Autodesk Inventor part; units mm, degrees
ref_plane "YZ Plane" through (0, 0, 0) normal (1, 0, 0) x (0, 1, 0)
ref_plane "XZ Plane" through (0, 0, 0) normal (0, 1, 0) x (-1, 0, 0)
ref_plane "XY Plane" through (0, 0, 0) normal (0, 0, 1) x (1, 0, 0)
sketch "Sketch1" plane through (0, 0, 0) normal (0, 0, 1) x (1, 0, 0)
  line L0 (0, 0) -> (90, 0)
  line L1 (90, 0) -> (90, 60)
  line L2 (90, 60) -> (0, 60)
  line L3 (0, 60) -> (0, 0)
  line L4 (-10, 30) -> (100, 30)
  line L5 (8, 10) -> (8, 50)
  line L6 (14, 10) -> (14, 50)
  arc A0 (14, 50) -> (8, 50) centre (11, 50) ccw
  arc A1 (8, 10) -> (14, 10) centre (11, 10) ccw
  arc A2 (22.5, 50) -> (16.5, 50) centre (19.5, 50) ccw
  line L7 (16.5, 10) -> (16.5, 50)
  line L8 (22.5, 10) -> (22.5, 50)
  arc A3 (16.5, 10) -> (22.5, 10) centre (19.5, 10) ccw
  arc A4 (31, 50) -> (25, 50) centre (28, 50) ccw
  line L9 (25, 10) -> (25, 50)
  line L10 (31, 10) -> (31, 50)
  arc A5 (25, 10) -> (31, 10) centre (28, 10) ccw
  arc A6 (39.5, 50) -> (33.5, 50) centre (36.5, 50) ccw
  line L11 (33.5, 10) -> (33.5, 50)
  line L12 (39.5, 10) -> (39.5, 50)
  arc A7 (33.5, 10) -> (39.5, 10) centre (36.5, 10) ccw
  arc A8 (48, 50) -> (42, 50) centre (45, 50) ccw
  line L13 (42, 10) -> (42, 50)
  line L14 (48, 10) -> (48, 50)
  arc A9 (42, 10) -> (48, 10) centre (45, 10) ccw
  arc A10 (56.5, 50) -> (50.5, 50) centre (53.5, 50) ccw
  line L15 (50.5, 10) -> (50.5, 50)
  line L16 (56.5, 10) -> (56.5, 50)
  arc A11 (50.5, 10) -> (56.5, 10) centre (53.5, 10) ccw
  line L17 (0, 60) -> (-6, 60)
  line L18 (-6, 60) -> (-6, 54)
  line L19 (-6, 54) -> (0, 48)
  line L20 (0, 0) -> (-6, 0)
  line L21 (-6, 0) -> (-6, 6)
  line L22 (-6, 6) -> (0, 12)
  line L23 (90, 60) -> (96, 60)
  line L24 (96, 60) -> (96, 54)
  line L25 (96, 54) -> (90, 48)
  line L26 (90, 0) -> (96, 0)
  line L27 (96, 0) -> (96, 6)
  line L28 (96, 6) -> (90, 12)
  circle A12 centre (3, 57) radius 1.65
  circle A13 centre (-3, 57) radius 1.65
  line L29 (45, 72.0135) -> (45, -11.3556)
  circle A14 centre (93, 57) radius 1.65
  circle A15 centre (-3, 3) radius 1.65
  circle A16 centre (93, 3) radius 1.65
  circle A17 centre (87, 57) radius 1.65
  circle A18 centre (3, 3) radius 1.65
  circle A19 centre (87, 3) radius 1.65
  arc A20 (65, 50) -> (59, 50) centre (62, 50) ccw
  line L30 (59, 10) -> (59, 50)
  line L31 (65, 10) -> (65, 50)
  arc A21 (59, 10) -> (65, 10) centre (62, 10) ccw
  arc A22 (73.5, 50) -> (67.5, 50) centre (70.5, 50) ccw
  line L32 (67.5, 10) -> (67.5, 50)
  line L33 (73.5, 10) -> (73.5, 50)
  arc A23 (67.5, 10) -> (73.5, 10) centre (70.5, 10) ccw
  arc A24 (82, 50) -> (76, 50) centre (79, 50) ccw
  line L34 (76, 10) -> (76, 50)
  line L35 (82, 10) -> (82, 50)
  arc A25 (76, 10) -> (82, 10) centre (79, 10) ccw
  dimension "d0" = 90
  dimension "d1" = 60
  dimension "d2" = 110
  dimension "d3" = 60
  dimension "d4" = 10
  dimension "d5" = 8
  dimension "d6" = 6
  dimension "d7" = 40
  dimension "d8" = 40
  dimension "d9" = 10
  dimension "d10" = 10
  dimension "d13" = 8.5
  dimension "d18" = 6
  dimension "d19" = 6
  dimension "d20" = 6
  dimension "d21" = 6
  dimension "d22" = 6
  dimension "d23" = 6
  dimension "d24" = 6
  dimension "d25" = 6
  dimension "d26" = 6
  dimension "d27" = 6
  dimension "d28" = 6
  dimension "d29" = 6
  dimension "d30" = 3.3
  dimension "d31" = 3.3
  dimension "d32" = 3
  dimension "d33" = 3
  dimension "d34" = 90
  dimension "d37" = 96
  dimension "d40" = 54
  dimension "d43" = 3
  dimension "d44" = 3
  dimension "d47" = 84
  dimension "d50" = 54
extrude "Extrusion1" add sketch "Sketch1" along normal blind 1.6 contours L3 L4 L5 A1 L6 L7 A3 L8 L9 A5 L10 L11 A7 L12 L13 A9 L29 L0 | L20 L21 L22 L3 | L29 A9 L14 L4 L15 A11 L16 L30 A21 L31 L32 A23 L33 L34 A25 L35 L1 L0 | L1 L28 L27 L26 | L3 L2 L29 A8 L13 L4 L12 A6 L11 L10 A4 L9 L8 A2 L7 L6 A0 L5 | L19 L18 L17 L3 | L4 L35 A24 L34 L33 A22 L32 L31 A20 L30 L16 A10 L15 L14 A8 L29 L2 L1 | L1 L23 L24 L25
sketch "Sketch2" plane through (0, 0, 1.6) normal (0, 0, 1) x (1, 0, 0)
  line L0 (96, 60) -> (-6, 60)
  line L1 (0, 0) -> (90, 0)
  line L2 (90, 0) -> (90, 60)
  line L3 (90, 60) -> (0, 60)
  line L4 (0, 60) -> (0, 0)
  line L5 (6, 5) -> (84, 5)
  line L6 (84, 5) -> (84, 55)
  line L7 (84, 55) -> (6, 55)
  line L8 (6, 55) -> (6, 5)
  circle A0 centre (3, 3) radius 1.65
  circle A1 centre (3, 3) radius 1.65
  circle A2 centre (3, 57) radius 1.65
  circle A3 centre (3, 57) radius 1.65
  circle A4 centre (87, 57) radius 1.65
  circle A5 centre (87, 57) radius 1.65
  circle A6 centre (87, 3) radius 1.65
  circle A7 centre (87, 3) radius 1.65
  point P0 (0, 60)
  dimension "d55" = 90
  dimension "d56" = 78
  dimension "d57" = 50
  dimension "d58" = 5
  dimension "d59" = 6
extrude "Extrusion2" add sketch "Sketch2" along normal blind 4
properties part number "IntakeFilterTop" material "PBT Plastic"
Input: part model. Units: mm. Frame: model coordinates. A direction names the side the tool comes from. Give positions to 0.01 mm unless a question says otherwise; leave off trailing zeros. Write each loop counter-clockwise with the first axis right and the second up, starting at its lowest first coordinate (ties: lowest second). Pieces come first, ordered by that corner, then holes. Notation, with made-up numbers: (-4, -26.75) - (20, -26.75) arc R17 cw to (20, -5.75) - close; hole circle Ø11 at (64.25, 13). An arc over 180 degrees is marked (long way). Write item = value, one per line. Start each with the question number.
1) Cut plane D-D (y = 38.5). Give the number of separate pieces and of enclosed holes in the cut face, and give its area (3 significant figures).
2) Material intervals for L1, parallel to Y at x = 87, z = 4.25; L2, parallel to X at y = 25, z = 2.85; L3, parallel to Y at x = 86, z = 1.65, sorted ascending. Write a range as [from, to].
3) Reachability of faces 3 (the face through (53.6, 7, 0.8)), 4 (the face through (33, 28, 1.6)), 5 (the face through (92, 5, 1.6)), 6 (the face through (90, 30, 3)), 7 (the face through (0, 30, 3)) from +Z, -Z, +X, -X, +Y, -Y: full face, straight path, thin tool, end or side. Return the list, or none.
4) Cut plane C-C (y = 57). Return loops of the section in (x, z).
5) Draft query along Y for faces 1 (the face through (1.69, 58, 2.76)), 2 (the face through (-2, 55, 1.6)). Return one class per face: pulls with the +Y half, pulls with the -Y half, needs draft (parallel to the pull), parting line crosses it, or undercut.
6) Cut plane A-A (x = 70.5). Return loops of the section in (y, z), and give its area (3 significant figures).
7) Pin query (flat end, axial travel): pin 1 (0.8 mm diameter, centred on y = 30.5, z = 0.5, fed in from +X); pin 2 (3 mm diameter, centred on x = 93, y = 3, fed in from +Z) (3 decimals); pin 3 (12 mm diameter, centred on x = 71.5, y = 20, fed in from +Z); pin 4 (1.8 mm diameter, centred on y = 33, z = 1, fed in from -X). Return the tip coordinate at first contact, or that it passes through.
8) Cut plane B-B (z = 3.5). Return loops of the section in (x, y).
Answers follow:
q1.separate_pieces = 10
q1.enclosed_holes = 0
q1.area = 106 mm^2
q2.L1 = [0, 1.35], [4.65, 55.35], [58.65, 60]
q2.L2 = [0, 6], [84, 90]
q2.L3 = [0, 1.69], [4.31, 55.69], [58.31, 60]
q3.face_3 = +Z, -Z
q3.face_4 = +Z
q3.face_5 = +Z, +X, +Y, -Y
q3.face_6 = +Z, +X
q3.face_7 = +Z, -X
q4.outline = (-6, 0) - (-4.65, 0) - (-4.65, 1.6) - (-6, 1.6) - close; (-1.35, 0) - (1.35, 0) - (1.35, 5.6) - (0, 5.6) - (0, 1.6) - (-1.35, 1.6) - close; (4.65, 0) - (85.35, 0) - (85.35, 5.6) - (4.65, 5.6) - close; (88.65, 0) - (91.35, 0) - (91.35, 1.6) - (90, 1.6) - (90, 5.6) - (88.65, 5.6) - close; (94.65, 0) - (96, 0) - (96, 1.6) - (94.65, 1.6) - close
q5.face_1 = undercut
q5.face_2 = needs draft
q6.outline = (0, 0) - (7, 0) - (7, 1.6) - (5, 1.6) - (5, 5.6) - (0, 5.6) - close; (53, 0) - (60, 0) - (60, 5.6) - (55, 5.6) - (55, 1.6) - (53, 1.6) - close
q6.area = 62.4 mm^2
q7.pin_1 = 90
q7.pin_2 = through
q7.pin_3 = 1.6
q7.pin_4 = 0
q8.outline = (0, 0) - (90, 0) - (90, 60) - (0, 60) - close; hole circle Ø3.3 at (3, 3); hole circle Ø3.3 at (3, 57); hole (6, 5) - (84, 5) - (84, 55) - (6, 55) - close; hole circle Ø3.3 at (87, 3); hole circle Ø3.3 at (87, 57)
